Model file for the job. Use its own axes, mm. Coordinates: 2 decimals unless noted, no trailing zeros. Write each loop counter-clockwise with the first axis right and the second up, starting at its lowest first coordinate (ties: lowest second). Pieces come first, ordered by that corner, then holes.
Q1. Band-saw the part on D-D, the plane z = 11.75. Write the cut outline in (x, y), plus the area to 3 significant figures.
Q2. Pin check, flat tips, straight feed: P1, Ø1, axis at y = 100.5, z = 10, coming from the -X side; P2, Ø1.5, axis at y = 392, z = 2, coming from the -X side; P3, Ø4, axis at y = 335.5, z = 2.5, coming from the -X side. Stop position of each tip, or through.
Q3. Drill centre lines: probe 1 along Y at (x, z) = (140, 12); probe 2 along Y at (x, z) = (138, 13.5); probe 3 along X at (y, z) = (323.5, 10.25). Where is each one in solid material? Low to high.
Q4. Band-saw the part on B-B, the plane x = 140. Write the cut outline in (y, z).
from build123d import *

# Parameters (mm, degrees)
SKETCH1_W           = 180
SKETCH1_H           = 480
SKETCH1_R           = 18.368726539
BOSS_EXTRUDE1_DEPTH = 18
CHAMFER1_SIZE       = 18


with BuildPart() as part:
    # Sketch1 → Boss-Extrude1 (new body)
    with BuildSketch(Plane.XY):
        with Locations((90, 240)):
            Rectangle(SKETCH1_W, SKETCH1_H)
        with Locations((140, 240)):
            Circle(SKETCH1_R, mode=Mode.SUBTRACT)
    extrude(amount=BOSS_EXTRUDE1_DEPTH)

    # Chamfer1
    chamfer1_edges = [part.edges().sort_by_distance(p)[0] for p in [
        (0, 240, 0),
    ]]
    chamfer(chamfer1_edges, length=CHAMFER1_SIZE - 0.0001)  # a hair under: the kernel refuses the full size


solid = part.part
Answer sheet:
1. outline: (6.25, 0) - (180, 0) - (180, 480) - (6.25, 480) - close; hole circle Ø36.74 at (140, 240)
1. area: 82,300 mm2
2. P1: stops at x = 7.5
2. P2: stops at x = 15.25
2. P3: stops at x = 13.5
3. probe 1: y = 0 to 221.63, 258.37 to 480
3. probe 2: y = 0 to 221.74, 258.26 to 480
3. probe 3: x = 7.75 to 180
4. outline: (0, 0) - (221.63, 0) - (221.63, 18) - (0, 18) - close; (258.37, 0) - (480, 0) - (480, 18) - (258.37, 18) - close
